Can you work these out from the model? Positions are in its coordinate system, mm. A direction names the side the tool comes from. Give positions to 0.01 mm unless a question says otherwise; leave off trailing zeros. Write each loop counter-clockwise with the first axis right and the second up, starting at its lowest first coordinate (ties: lowest second). Pieces come first, ordered by that corner, then holes. Notation, with made-up numbers: M -24.5,10.5 L -12.5,10.5 A29 cw -12.5,49.5 Z; hole C 84.5,54 d9. An arc over 180 degrees is marked long. Write each question's results on one line, items separated by ' | '.
from build123d import *

# Parameters (mm, degrees)
F1_DEPTH = 5
F2_R     = 1.5
F3_DEPTH = 12.5
F5_R     = 3
F6_R     = 3
F7_DEPTH = 25


with BuildPart() as f1:
    # F0 (on Front) → F1 (new body, symmetric)
    with BuildSketch(Plane.XZ):
        with BuildLine():
            ThreePointArc((2, 40.35103), (0, 13.5), (-2, 40.35103))
            Line((-2, 40.35103), (-2, 40.404946))
            Line((-2, 40.404946), (-2, 50.35103))
            Line((-2, 50.35103), (-6, 50.35103))
            Line((-6, 50.35103), (-6, 43.970563))
            ThreePointArc((-6, 43.970563), (-14.696938, 37.392305), (-18, 27))
            Line((-18, 27), (-18, 5))
            Line((-18, 5), (-32.5, 5))
            Line((-32.5, 5), (-32.5, 0))
            Line((-32.5, 0), (-15, 0))
            Line((-15, 0), (15, 0))
            Line((15, 0), (32.5, 0))
            Line((32.5, 0), (32.5, 5))
            Line((32.5, 5), (18, 5))
            Line((18, 5), (18, 27))
            ThreePointArc((18, 27), (14.696938, 37.392305), (6, 43.970563))
            Line((6, 43.970563), (6, 50.35103))
            Line((6, 50.35103), (2, 50.35103))
            Line((2, 50.35103), (2, 40.35103))
        make_face()
    extrude(amount=F1_DEPTH, both=True)


with BuildPart() as f3:
    # F2 (on Right) → F3 (new body, symmetric)
    with BuildSketch(Plane.YZ):
        with Locations((0, 47)):
            Circle(F2_R)
    extrude(amount=F3_DEPTH, both=True)


with BuildPart() as f1_1:
    add(f1.part)

    # F4: cut F3
    add(f3.part, mode=Mode.SUBTRACT)

    # F5
    f5_edges = [f1_1.edges().sort_by_distance(p)[0] for p in [
        (18, 0, 5),
        (-18, 0, 5),
    ]]
    fillet(f5_edges, radius=F5_R)


with BuildPart() as f7:
    # F6 (on Top) → F7 (new body)
    with BuildSketch(Plane.XY):
        with Locations((-25, 0)):
            Circle(F6_R)
        with Locations((25.418336, 0)):
            Circle(F6_R)
    extrude(amount=F7_DEPTH)


with BuildPart() as f1_2:
    add(f1_1.part)

    # F8: cut F7
    add(f7.part, mode=Mode.SUBTRACT)


solid = f1_2.part
Item 1: I want a section at C-C, the plane x = -3.5. Please give me the cut outline in (y, z), and give its area (3 significant figures).
Geometry says:
outline: M -5,0 L 5,0 L 5,13.96 L -5,13.96 Z; M -5,40.04 L 5,40.04 L 5,50.35 L -5,50.35 Z; hole C 0,47 d3 | area: 236 mm2
Item 2: I'm going to push flat-ended pins straight in: pin 1 (1.5 mm diameter, centred on x = -7, y = 2.5, fed in from +Z); pin 2 (3 mm diameter, centred on y = -1.5, z = 19.5, fed in from +X); pin 3 (5 mm diameter, centred on y = -0.5, z = 47, fed in from -X). Where does each tip first touch, or does it pass through?
Geometry says:
pin 1: stops at z = 43.88 | pin 2: stops at x = 18 | pin 3: stops at x = -6
Item 3: Thinking about a two-plate mould opening in Y: for faces 1 (the face through (22.42, 0.13, 2.46)), 2 (the face through (0, -5, 12)), 3 (the face through (6, 0, 49)), which applies, +Y half, -Y half, draft (parallel to the pull), parting line (faces both ways), or undercut?
Geometry says:
face 1: undercut | face 2: -Y half | face 3: draft
Item 4: I want a section at A-A, the plane y = 0. Give the number of separate pieces and of enclosed holes in the cut face, and give its area (3 significant figures).
Geometry says:
separate pieces: 5 | enclosed holes: 0 | area: 1,000 mm2
Item 5: For faces 4 (the face through (-6, 0, 49)), 5 (the face through (-28, 0, 2)), 6 (the face through (2, 0, 45)), 7 (the face through (18, 0, 17)), which set-ups out of +Z, -Z, +X, -X, +Y, -Y let a thin tool reach every point of the face, with its end or its side?
Geometry says:
face 4: +Z, -X, +Y, -Y | face 5: +Z, -Z | face 6: +Z, +Y, -Y | face 7: +Z, +X, +Y, -Y
Item 6: If I drill on line 1 (X direction, y = 0, z = 2.95); line 2 (X direction, y = -2.5, z = 27); line 3 (Y direction, x = -25, z = 1.35), over which ranges is the centre line in solid material (lowest first)? Write a range as from..to.
Geometry says:
line 1: x = -32.5..-28, -22..22.42, 28.42..32.5 | line 2: x = -18..-13.5, 13.5..18 | line 3: y = -5..-3, 3..5
Item 7: I want a section at D-D, the plane x = 12. Please give me the cut outline in (y, z), and give its area (3 significant figures).
Geometry says:
outline: M -5,0 L 5,0 L 5,20.82 L -5,20.82 Z; M -5,33.18 L 5,33.18 L 5,40.42 L -5,40.42 Z | area: 280 mm2
Item 8: I want a section at B-B, the plane z = 47. Please give me the cut outline in (x, y).
Geometry says:
outline: M -6,-5 L -2,-5 L -2,-1.5 L -6,-1.5 Z; M -6,1.5 L -2,1.5 L -2,5 L -6,5 Z; M 2,-5 L 6,-5 L 6,-1.5 L 2,-1.5 Z; M 2,1.5 L 6,1.5 L 6,5 L 2,5 Z
